from build123d import *

# Parameters (mm, degrees)
BOSS_EXTRUDE1_DEPTH = 19.05
SKETCH2_R           = 3.81
CUT_EXTRUDE1_DEPTH  = 77.2
SKETCH3_R           = 3.81
CUT_EXTRUDE2_DEPTH  = 20.05
CHAMFER1_SIZE       = 2.54


with BuildPart() as part:
    # Sketch1 → Boss-Extrude1 (new body)
    with BuildSketch(Plane(origin=(0, 0, 0), x_dir=(0, 0, -1), z_dir=(1, 0, 0))):
        with BuildLine():
            Line((50.8, 0), (50.8, 30.48))
            ThreePointArc((50.8, 30.48), (54.048946048, 51.76907936), (63.5, 71.12))
            Line((63.5, 71.12), (63.5, 127))
            Line((63.5, 127), (38.1, 127))
            Line((38.1, 127), (38.1, 101.6))
            Line((38.1, 101.6), (12.7, 101.6))
            Line((12.7, 101.6), (12.7, 127))
            Line((12.7, 127), (-12.7, 127))
            Line((-12.7, 127), (-12.7, 71.12))
            ThreePointArc((-12.7, 71.12), (-3.248946048, 51.76907936), (0, 30.48))
            Line((0, 30.48), (0, 0))
            Line((0, 0), (50.8, 0))
        make_face()
    extrude(amount=BOSS_EXTRUDE1_DEPTH)

    # Sketch2 → Cut-Extrude1 (cut, through all)
    with BuildSketch(Plane.XY.offset(12.7)):
        with Locations((9.525, 116.84)):
            Circle(SKETCH2_R)
        with Locations((9.525, 91.44)):
            Circle(SKETCH2_R)
        with Locations((9.525, 10.16)):
            Circle(SKETCH2_R)
    extrude(amount=-CUT_EXTRUDE1_DEPTH, mode=Mode.SUBTRACT)

    # Sketch3 → Cut-Extrude2 (cut, through all)
    with BuildSketch(Plane(origin=(19.05, 0, 0), x_dir=(0, 0, -1), z_dir=(1, 0, 0))):
        with Locations((25.4, 50.8)):
            Circle(SKETCH3_R)
    extrude(amount=-CUT_EXTRUDE2_DEPTH, mode=Mode.SUBTRACT)

    # Chamfer1
    chamfer1_edges = [part.edges().sort_by_distance(p)[0] for p in [
        (0, 127, 0),
        (0, 127, -50.8),
        (0, 0, -25.4),
        (19.05, 127, -50.8),
        (19.05, 127, 0),
        (19.05, 0, -25.4),
    ]]
    chamfer(chamfer1_edges, length=CHAMFER1_SIZE)


solid = part.part
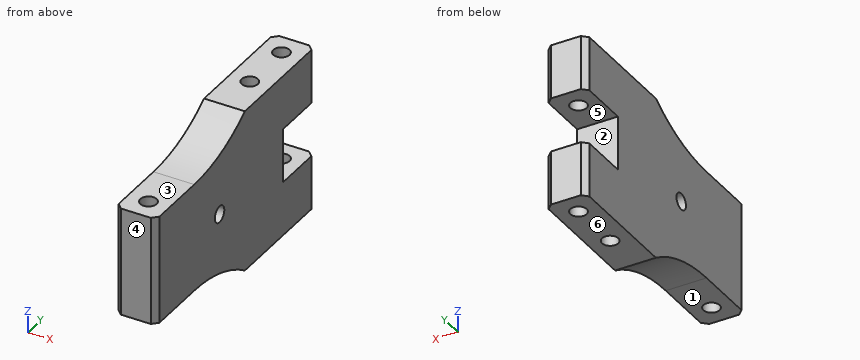
The model under review builds one solid part; all positions refer to its coordinate system, in mm. Face numbers are marked on the shaded views. A direction names the side the tool comes from. Give positions to 0.01 mm unless a question says otherwise; leave off trailing zeros. Order: outer loops, then holes, each group sorted by start corner. A loop starts at its lowest first (then second) coordinate and runs counter-clockwise, first axis right, second up. Notation, with made-up numbers: M 88.5,78 L 115.5,78 A9 cw 115.5,84 Z; hole C -13.5,21.5 d2. An arc over 180 degrees is marked long. Answer in a Markdown table with one row per item. Add a question column.
1. For pin 1 Ø7 at (x, y) = (9.525, 116.84) entering from -Z; pin 2 Ø8 at (x, y) = (2.5, 69.5) entering from +Z; pin 3 Ø9.5 at (x, y) = (5, 19.5) entering from -Z; pin 4 Ø9.5 at (x, z) = (7, -30.5) entering from +Y, all flat-tipped, find the tip position at first contact; note any pin that passes through.
2. Add section A-A on z = -25.4. State the section outline as (x, y) points (3 decimals).
3. Machinability: for the marked faces 1, 2 and 3, which of the approach directions +Z, -Z, +X, -X, +Y, -Y give a long, thin tool a straight path to every point of the face, cutting with its end or side? Answer none if there is none.
4. Add section C-C on y = 10.16. State the section outline as (x, z) points (3 decimals), plus the area to 3 significant figures.
5. Add section B-B on y = 116.84. State the section outline as (x, z) points (3 decimals).
6. To check wall thickness, follow line 1 along Y through (x, z) = (8.5, -21.5); line 2 along Y through (x, z) = (9.5, -26); line 3 along X through (y, z) = (117, 2.5). State the ranges of each line that lie inside material, in increasing order.
7. Mouldability with a two-part tool opening along Z and no side actions: class the marked faces 4, 5 and 6 as released by +Z, released by -Z, zero draft, split by the parting line, or undercut.
8. Add section D-D on z = -35. State the section outline as (x, y) points (3 decimals).
The answers:
| question | item | result |
|---|---|---|
| 1 | pin 1 | through |
| 1 | pin 2 | z = 12.7 |
| 1 | pin 3 | z = -50.8 |
| 1 | pin 4 | y = 101.6 |
| 2 | outline | M 0,2.54 L 2.54,0 L 16.51,0 L 19.05,2.54 L 19.05,46.99 L 0,46.99 Z; M 0,54.61 L 19.05,54.61 L 19.05,101.6 L 0,101.6 Z; hole C 9.525,10.16 d7.62; hole C 9.525,91.44 d7.62 |
| 3 | face 1 | -Z, +X, -X, -Y |
| 3 | face 2 | +X, -X, +Y |
| 3 | face 3 | +Z, +X, -X, -Y |
| 4 | outline | M 0,-50.8 L 5.715,-50.8 L 5.715,0 L 0,0 Z; M 13.335,-50.8 L 19.05,-50.8 L 19.05,0 L 13.335,0 Z |
| 4 | area | 581 mm2 |
| 5 | outline | M 0,-63.5 L 5.715,-63.5 L 5.715,-38.1 L 0,-38.1 Z; M 0,-12.7 L 5.715,-12.7 L 5.715,12.7 L 0,12.7 Z; M 13.335,-63.5 L 19.05,-63.5 L 19.05,-38.1 L 13.335,-38.1 Z; M 13.335,-12.7 L 19.05,-12.7 L 19.05,12.7 L 13.335,12.7 Z |
| 6 | line 1 | 0 to 6.49, 13.83 to 87.77, 95.11 to 101.6 |
| 6 | line 2 | 0 to 6.35, 13.97 to 47.04, 54.56 to 87.63, 95.25 to 101.6 |
| 6 | line 3 | 0 to 5.72, 13.33 to 19.05 |
| 7 | face 4 | zero draft |
| 7 | face 5 | undercut |
| 7 | face 6 | released by -Z |
| 8 | outline | M 0,2.54 L 2.54,0 L 16.51,0 L 19.05,2.54 L 19.05,101.6 L 0,101.6 Z; hole C 9.525,10.16 d7.62; hole C 9.525,91.44 d7.62 |
